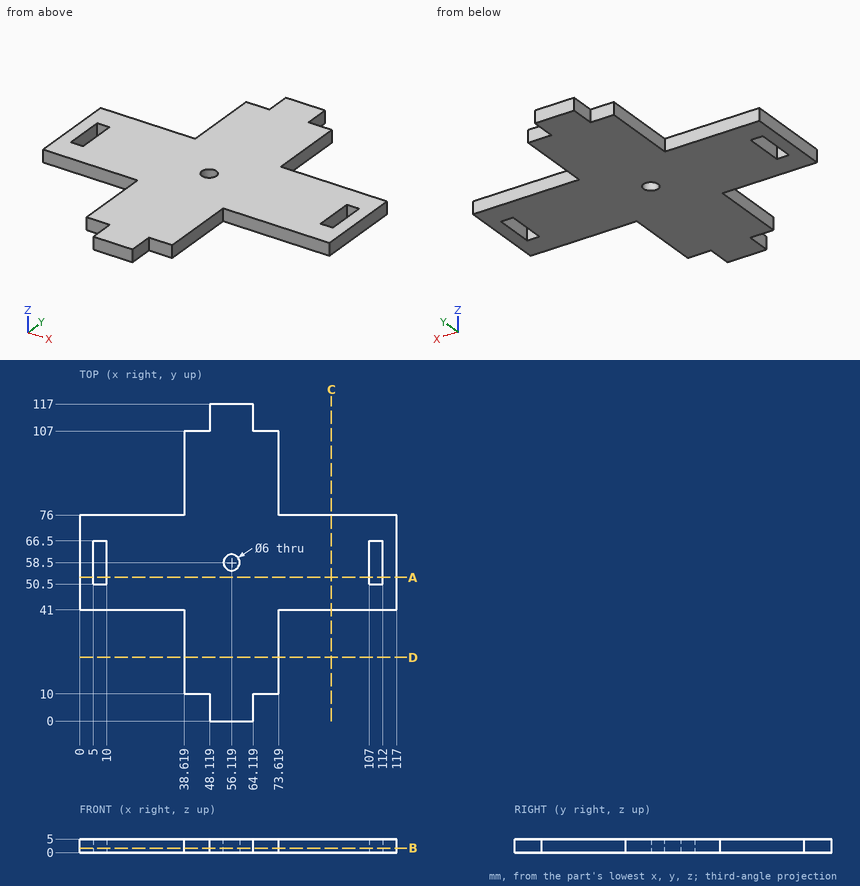
Answer from the drawing. Dimensions are ordinates in mm from the lowest x, y and z of the part. Round coordinates to 2 decimals unless told otherwise and drop trailing zeros. Loops run counter-clockwise (first coordinate to the right, second up) from the corner with the lowest first, then second, coordinate; pieces in that order, holes last. Notation, with made-up numbers: M 89,78.25 L 97,78.25 A13 cw 97,91.25 Z; hole C -9.75,-8.5 d8. An arc over 180 degrees is marked long. One line per question, with ' | ' between items. Start each with the question number.
(1) Find the intervals of material crossed by line 1 (Y direction, x = 56.5, z = 1.35) (1 decimal); line 2 (X direction, y = 10.5, z = 3.2); line 3 (Y direction, x = 97, z = 0.85), in increasing order.
(2) A cutting plane is placed at C-C on x = 93. Write down the section's boundary in (y, z).
(3) A cutting plane is placed at D-D on y = 23.5. Write down the section's boundary in (x, z), plus the area to 3 significant figures.
(4) A cutting plane is placed at A-A on y = 53. Write down the section's boundary in (x, z), plus the area to 3 significant figures.
(5) Flat-ended cylindrical pins translate along their axes: pin 1 Ø1.5 at (x, z) = (92, 3.5) entering from -Y; pin 2 Ø2.5 at (x, z) = (102.5, 3) entering from +Y; pin 3 Ø2.5 at (x, z) = (68.5, 2.5) entering from -Y. Find the tip coordinate at first contact, or state that the pin passes through.
(6) A cutting plane is placed at B-B on z = 1.6. Give the number of separate pieces and of enclosed holes in the cut face, plus the area to 3 significant figures.
Geometry check:
1) line 1: y = 0 to 55.5, 61.5 to 117 | line 2: x = 38.62 to 73.62 | line 3: y = 41 to 76
2) outline: M 41,0 L 76,0 L 76,5 L 41,5 Z
3) outline: M 38.62,0 L 73.62,0 L 73.62,5 L 38.62,5 Z | area: 175 mm²
4) outline: M 0,0 L 5,0 L 5,5 L 0,5 Z; M 10,0 L 107,0 L 107,5 L 10,5 Z; M 112,0 L 117,0 L 117,5 L 112,5 Z | area: 535 mm²
5) pin 1: stops at y = 41 | pin 2: stops at y = 76 | pin 3: stops at y = 10
6) separate pieces: 1 | enclosed holes: 3 | area: 6,400 mm²
